Here's the drawing with two shaded views (mm, measured from the low corner). I have some questions. Round coordinates to 2 decimals unless told otherwise and drop trailing zeros. Order: outer loops, then holes, each group sorted by start corner. A loop starts at its lowest first (then second) coordinate and runs counter-clockwise, first axis right, second up. Notation, with made-up numbers: (54, 6.5) -> (101, 6.5) arc R9 cw to (101, 13.5) -> close; hole circle Ø1 at (5.25, 42.5). An arc over 180 degrees is marked (long way). Use a Markdown table: item, result. Add a question column.
Q1. We'd pull the mould along X, two halves only. Please class the marked faces 1, 2 and 3: +X half, -X half, draft (parallel to the pull), parting line (faces both ways), or undercut.
Q2. If we section it at D-D on y = 148.5: List the corners of the cut face in (x, z) for me.
Q3. I'm going to push flat-ended pins straight in: pin 1 Ø12 at (y, z) = (355, 233.5) entering from -X; pin 2 Ø3 at (y, z) = (518.5, 81.5) entering from -X; pin 3 Ø12 at (x, z) = (201, 87.5) entering from +Y. Where does each tip first touch, or does it pass through?
Q4. If we section it at A-A on y = 300: List the corners of the cut face in (x, z) for me.
Q5. If we section it at C-C on z = 60: List the corners of the cut face in (x, y) for me, plus the area to 3 significant figures.
Q6. I need wall thicknesses on line 1 along Y through (x, z) = (300, 295.75); line 2 along Y through (x, z) = (300, 127); line 3 along Z through (x, y) = (201, 409). Which ranges of each line are inside material? Lowest first, please. Write a range as [from, to].
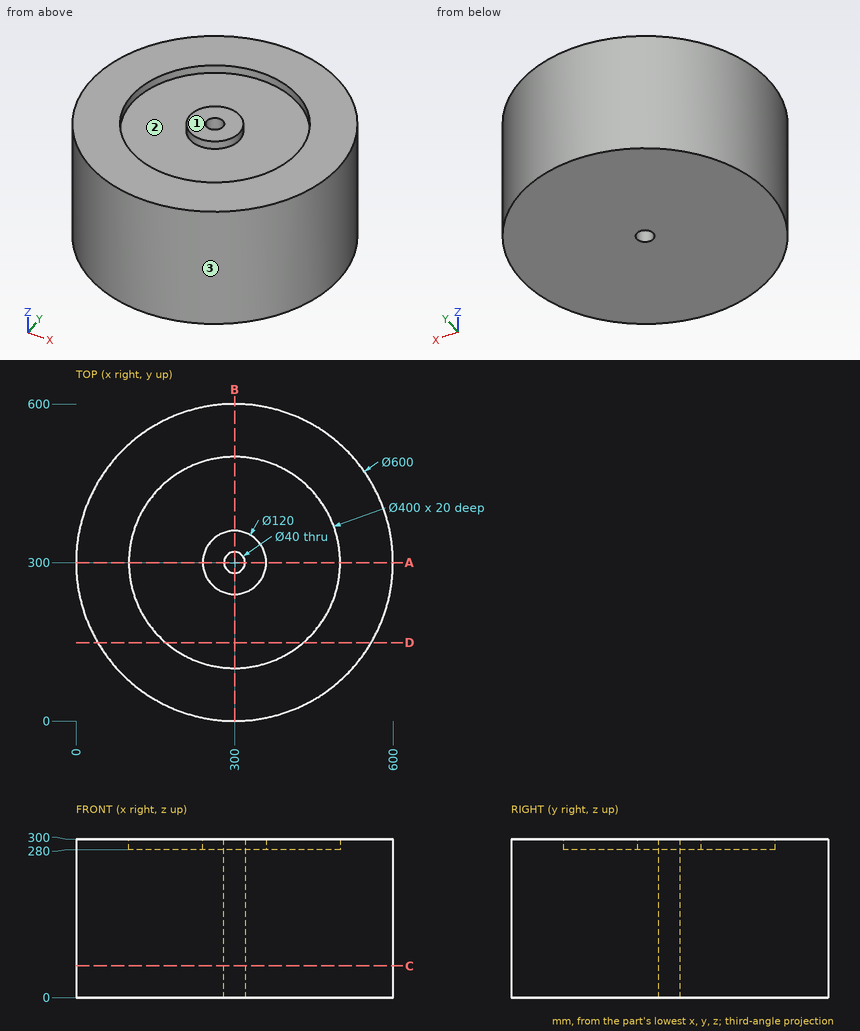
Answer below:
| question | item | result |
|---|---|---|
| 1 | face 1 | draft |
| 1 | face 2 | undercut |
| 1 | face 3 | parting line |
| 2 | outline | (41.06, 0) -> (558.94, 0) -> (558.94, 300) -> (430.57, 300) -> (430.57, 280) -> (169.43, 280) -> (169.43, 300) -> (41.06, 300) -> close |
| 3 | pin 1 | x = 4.03 |
| 3 | pin 2 | x = 92.85 |
| 3 | pin 3 | y = 585.22 |
| 4 | outline | (0, 0) -> (280, 0) -> (280, 300) -> (240, 300) -> (240, 280) -> (100, 280) -> (100, 300) -> (0, 300) -> close; (320, 0) -> (600, 0) -> (600, 300) -> (500, 300) -> (500, 280) -> (360, 280) -> (360, 300) -> (320, 300) -> close |
| 5 | outline | circle Ø600 at (300, 300); hole circle Ø40 at (300, 300) |
| 5 | area | 281,000 mm² |
| 6 | line 1 | [0, 100], [240, 280], [320, 360], [500, 600] |
| 6 | line 2 | [0, 280], [320, 600] |
| 6 | line 3 | [0, 280] |
